Work out the finished part from the listing and answer in its coordinate system (mm). A direction names the side the tool comes from. Round coordinates to 2 decimals unless told otherwise and drop trailing zeros. Write each loop counter-clockwise with the first axis right and the second up, starting at its lowest first coordinate (ties: lowest second). Pieces come first, ordered by that corner, then holes.
1. Flat-ended cylindrical pins translate along their axes: pin 1 Ø5.5 at (y, z) = (24, 39) entering from -X; pin 2 Ø3 at (y, z) = (31.5, 16) entering from -X; pin 3 Ø3.5 at (y, z) = (14.5, 81.5) entering from -X; pin 4 Ø8 at (x, z) = (1.5, 34.5) entering from +Y. Find the tip coordinate at first contact, or state that the pin passes through.
2. Find section A-A (z = 4.5). Write down the section's boundary in (x, y), and give its area (3 significant figures).
3. Straight lines are drawn through the part: probe 1 along Z at (x, y) = (47, -23.5); probe 2 along Z at (x, y) = (76.5, -5.5); probe 3 along Z at (x, y) = (33, -31). For each, find the intervals that lie inside material, in ascending order.
4. Determine the mould class of faces 5 (the face through (-0.711, 61.972, 13.791)), 6 (the face through (-50.8, -1, 0)), 7 (the face through (1, -27, 15.24)) for opening direction Z: pulls with the +Z half, pulls with the -Z half, needs draft (parallel to the pull), parting line crosses it, or undercut.
5. Find section B-B (x = 80). Write down the section's boundary in (y, z), and give its area (3 significant figures).
6. A tool of negligible diameter and unlimited length cuts with its end or side. For faces 1 (the face through (85, 0, 54.698)), 2 (the face through (47, 25.4, 64)), 3 (the face through (29.9, -0.4, 58.9)), 4 (the face through (47, -25.4, 64)), from which of +Z, -Z, +X, -X, +Y, -Y can it reach the whole face along a straight path? Write none if from no direction.
```python
from build123d import *

# Parameters (mm, degrees)
F1_DEPTH = 63.5
F2_R     = 5.08
F0_W     = 23.8256007433
F0_H     = 15.24
F0_H_2   = 4.5536607504
F0_H_3   = 8.295490036
F3_DEPTH = 25.4
F4_DEPTH = 20.32


with BuildPart() as f1:
    # F0 (on Front) → F1 (new body, symmetric)
    with BuildSketch(Plane.XZ):
        Polygon((50.8, 15.24), (25.0475049125, 15.24), (9.811083613, 15.24), (-50.8, 15.24), (-50.8, -15.24), (50.8, -15.24), align=None)
    extrude(amount=F1_DEPTH, both=True)

    # F2
    f2_edges = [f1.edges().sort_by_distance(p)[0] for p in [
        (0, -63.5, 15.24),
        (50.8, -63.5, 0),
        (50.8, 63.5, 0),
        (-50.8, -63.5, 0),
        (-50.8, 63.5, 0),
        (0, 63.5, 15.24),
    ]]
    fillet(f2_edges, radius=F2_R)

    # F0 (on Front) → F3 (join, symmetric)
    with BuildSketch(Plane.XZ):
        with BuildLine():
            Line((9.811083613, 15.24), (25.0475049125, 15.24))
            Line((25.0475049125, 15.24), (25.0475049125, 49.1612727198))
            ThreePointArc((25.0475049125, 49.1612727198), (30.0363393946, 59.0226161714), (40.349945426, 62.9930185175))
            Line((40.349945426, 62.9930185175), (60.413621366, 62.9930185175))
            Line((60.413621366, 62.9930185175), (60.413621366, 78.2330185175))
            Line((60.413621366, 78.2330185175), (40.349945426, 78.2330185175))
            ThreePointArc((40.349945426, 78.2330185175), (19.4853705585, 70.0242707851), (9.8075049125, 49.7992135472))
            Line((9.8075049125, 49.7992135472), (9.8075049125, 16.6551610548))
            Line((9.8075049125, 16.6551610548), (9.811083613, 15.24))
        make_face()
        with Locations((72.3264217377, 70.6130185175)):
            Rectangle(F0_W, F0_H)
        with Locations((72.3264217377, 80.5098488927)):
            Rectangle(F0_W, F0_H_2)
        with Locations((72.3264217377, 58.8452734995)):
            Rectangle(F0_W, F0_H_3)
    extrude(amount=F3_DEPTH, both=True)

    # F0 (on Front) → F4 (join, symmetric)
    with BuildSketch(Plane.XZ):
        with BuildLine():
            Line((-50.8, 15.24), (9.811083613, 15.24))
            Line((9.811083613, 15.24), (9.8075049125, 16.6551610548))
            Line((9.8075049125, 16.6551610548), (9.8075049125, 49.7992135472))
            ThreePointArc((9.8075049125, 49.7992135472), (19.4853705585, 70.0242707851), (40.349945426, 78.2330185175))
            add(Edge.make_bspline(
                [(-50.8, 15.24), (-50.6889559329, 50.4340007901), (-17.0823093504, 78.5231366754), (40.349945426, 78.2330185175)],
                knots=[0, 0, 0, 0, 110.7990655787, 110.7990655787, 110.7990655787, 110.7990655787], degree=3))
        make_face()
    extrude(amount=F4_DEPTH, both=True)

    # F0 (on Front) → F5 (revolve)
    with BuildSketch(Plane.XZ):
        Polygon((84.2392221093, 78.2330185175), (84.2392221093, 62.9930185175), (84.2392221093, 54.6975284815), (108.5664257407, 54.6975284815), (108.5664257407, 82.7866792679), (84.2392221093, 82.7866792679), align=None)
    revolve(axis=Axis((84.2392221093, 0, 68.7421038747), (0, 0, 1)))


solid = f1.part
```
Worked answers:
1. pin 1: stops at x = 9.81
1. pin 2: stops at x = -50.8
1. pin 3: stops at x = 60.41
1. pin 4: stops at y = 20.32
2. outline: (-50.8, -58.42) arc R5.08 ccw to (-45.72, -63.5) - (45.72, -63.5) arc R5.08 ccw to (50.8, -58.42) - (50.8, 58.42) arc R5.08 ccw to (45.72, 63.5) - (-45.72, 63.5) arc R5.08 ccw to (-50.8, 58.42) - close
2. area: 12,900 mm2
3. probe 1: z = -15.24 to 15.24, 62.99 to 78.23
3. probe 2: z = 54.7 to 82.79
3. probe 3: z = -15.24 to 15.24
4. face 5: pulls with the +Z half
4. face 6: needs draft
4. face 7: undercut
5. outline: (-25.4, 54.7) - (25.4, 54.7) - (25.4, 82.79) - (-25.4, 82.79) - close
5. area: 1,430 mm2
6. face 1: -Z, +X, +Y, -Y
6. face 2: +Z, +X, -X, +Y
6. face 3: +Y, -Y
6. face 4: +Z, +X, -X, -Y
